The drawing under review shows one solid part. Ordinate dimensions are in mm from its lowest x, y, z. A direction names the side the tool comes from. Coordinates: 2 decimals unless noted, no trailing zeros. Order: outer loops, then holes, each group sorted by start corner. A loop starts at its lowest first (then second) coordinate and runs counter-clockwise, first axis right, second up. Notation, with made-up numbers: (-18.75, 37) - (29.25, 37) arc R27 cw to (29.25, 71) - close; hole circle Ø2 at (89.5, 78.25). An arc over 180 degrees is marked (long way). Answer in a Markdown table with one row per item.
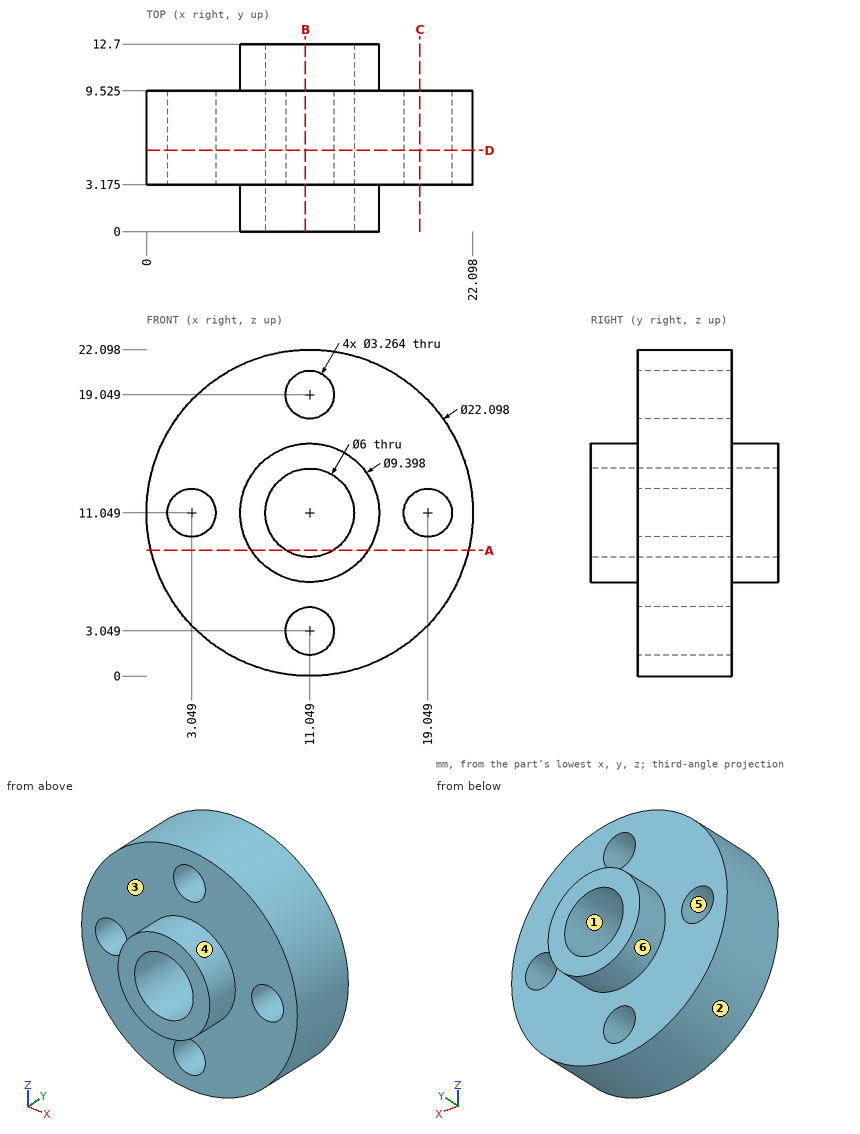
Item 1: Mouldability with a two-part tool opening along X and no side actions: class the marked faces 1, 2 and 3 as +X half, -X half, draft (parallel to the pull), parting line (faces both ways), or undercut.
Check values:
| item | result |
|---|---|
| face 1 | undercut |
| face 2 | parting line |
| face 3 | draft |
Item 2: We need section C-C, the plane x = 18.5. Write out the cut boundary in (y, z) (1 decimal), then the cut area to 3 significant figures.
Check values:
| item | result |
|---|---|
| outline | (3.2, 2.9) - (9.5, 2.9) - (9.5, 9.5) - (3.2, 9.5) - close; (3.2, 12.6) - (9.5, 12.6) - (9.5, 19.2) - (3.2, 19.2) - close |
| area | 84.1 mm^2 |
Item 3: Clearance check with flat-ended pins moving along their axes: pin 1 Ø1.5 at (x, z) = (17, 8.5) entering from -Y (3 decimals); pin 2 Ø3 at (x, y) = (8.5, 6) entering from +Z; pin 3 Ø4 at (x, z) = (11.049, 19.049) entering from +Y (3 decimals). State where each tip first meets the part, or that it passes through.
Check values:
| item | result |
|---|---|
| pin 1 | y = 3.175 |
| pin 2 | z = 22.05 |
| pin 3 | y = 9.525 |
Item 4: We need section B-B, the plane x = 10.75. Write out the cut boundary in (y, z) (1 decimal).
Check values:
| item | result |
|---|---|
| outline | (0, 6.4) - (3.2, 6.4) - (3.2, 4.7) - (9.5, 4.7) - (9.5, 6.4) - (12.7, 6.4) - (12.7, 8.1) - (0, 8.1) - close; (0, 14) - (12.7, 14) - (12.7, 15.7) - (9.5, 15.7) - (9.5, 17.4) - (3.2, 17.4) - (3.2, 15.7) - (0, 15.7) - close; (3.2, 0) - (9.5, 0) - (9.5, 1.4) - (3.2, 1.4) - close; (3.2, 20.7) - (9.5, 20.7) - (9.5, 22.1) - (3.2, 22.1) - close |
Item 5: We need section D-D, the plane y = 5.5. Write out the cut boundary in (x, z).
Check values:
| item | result |
|---|---|
| outline | circle Ø22.1 at (11.05, 11.05); hole circle Ø3.26 at (3.05, 11.05); hole circle Ø6 at (11.05, 11.05); hole circle Ø3.26 at (11.05, 3.05); hole circle Ø3.26 at (11.05, 19.05); hole circle Ø3.26 at (19.05, 11.05) |
Item 6: To check wall thickness, follow line 1 (Z direction, x = 11, y = 1.75); line 2 (Y direction, x = 7.75, z = 17.25) (3 decimals); line 3 (X direction, y = 5, z = 12) (1 decimal). State the ranges of each line that lie inside material, in increasing order. Write a range as from..to.
Check values:
| item | result |
|---|---|
| line 1 | 6.35..8.05, 14.05..15.75 |
| line 2 | 3.175..9.525 |
| line 3 | 0..1.7, 4.4..8.2, 13.9..17.7, 20.4..22.1 |
Item 7: We need section A-A, the plane z = 8.5. Write out the cut boundary in (x, y) (1 decimal), then the cut area to 4 significant figures.
Check values:
| item | result |
|---|---|
| outline | (0.3, 3.2) - (7.1, 3.2) - (7.1, 0) - (9.5, 0) - (9.5, 12.7) - (7.1, 12.7) - (7.1, 9.5) - (0.3, 9.5) - close; (12.6, 0) - (15, 0) - (15, 3.2) - (21.8, 3.2) - (21.8, 9.5) - (15, 9.5) - (15, 12.7) - (12.6, 12.7) - close |
| area | 146.5 mm^2 |
Item 8: Tool access review of the marked faces 4, 5 and 6: name each direction out of +Z, -Z, +X, -X, +Y, -Y from which nothing blocks a thin tool from reaching the whole face with its end or side.
Check values:
| item | result |
|---|---|
| face 4 | -Y |
| face 5 | +Y, -Y |
| face 6 | +Y |
